The listing builds one solid part. Answer for the finished solid, in the listing's coordinates (mm). A direction names the side the tool comes from. Coordinates: 2 decimals unless noted, no trailing zeros. Order: outer loops, then holes, each group sorted by start corner. A loop starts at its lowest first (then second) coordinate and runs counter-clockwise, first axis right, second up.
```python
from build123d import *

# Parameters (mm, degrees)
F0_W     = 351.6883096945
F0_H     = 200
F1_DEPTH = 25
F2_T     = -2.5
F4_DEPTH = 25


with BuildPart() as f1:
    # F0 (on Front) → F1 (new body)
    with BuildSketch(Plane.XZ):
        with Locations((-175.8441548473, 100)):
            Rectangle(F0_W, F0_H)
    extrude(amount=F1_DEPTH)

    # F2
    f2_openings = [f1.faces().sort_by_distance(p)[0] for p in [
        (-175.844155, -25, 100),
    ]]
    offset(amount=F2_T, openings=f2_openings)

    # F3 (on face) → F4 (join)
    with BuildSketch(Plane.XZ.offset(2.5)):
        Polygon((-291.9401824474, 119.7359256967), (-280.8749377728, 126.1244476883), (-291.9401824474, 132.5129696799), align=None)
        Polygon((-269.8096930981, 106.9588817135), (-269.8096930981, 119.7359256967), (-280.8749377728, 126.1244476883), (-291.9401824474, 119.7359256967), (-291.9401824474, 106.9588817135), (-280.8749377728, 100.570359722), align=None)
        Polygon((-269.8096930981, 119.7359256967), (-269.8096930981, 132.5129696799), (-280.8749377728, 126.1244476883), align=None)
        Polygon((-269.8096930981, 94.1818377304), (-269.8096930981, 106.9588817135), (-280.8749377728, 100.570359722), align=None)
        Polygon((-291.9401824474, 94.1818377304), (-280.8749377728, 100.570359722), (-291.9401824474, 106.9588817135), align=None)
        Polygon((-291.9401824474, 106.9588817135), (-291.9401824474, 119.7359256967), (-303.0054271221, 113.3474037051), align=None)
        Polygon((-258.7444484234, 113.3474037051), (-269.8096930981, 119.7359256967), (-269.8096930981, 106.9588817135), align=None)
    extrude(amount=F4_DEPTH)


solid = f1.part
```
1) Each of these flat-tipped pins is pushed along its axis until it touches: P1, Ø3, axis at x = -172, z = 166, coming from the -Y side; P2, Ø3, axis at x = -240, y = -8, coming from the -Z side. Where does it stop, or does it pass through?
2) A cutting plane is placed at B-B, the plane z = 183. Write down the section's boundary in (x, y), plus the area to 3 significant figures.
3) The mould has two halves that part along Z. Classify faces 3 (the flat face through (-178, -12, 200)), 4 (the flat face through (-291.94, -15, 126)), 5 (the flat face through (-178, 0, 101)): released by +Z, released by -Z, zero draft, split by the parting line, or undercut.
4) A cutting plane is placed at C-C, the plane x = -46. Write down the section's boundary in (y, z), plus the area to 4 significant figures.
5) For faces 1 (the flat face through (-351.688, -12, 99)), 2 (the flat face through (-275.42, -14.82, 97.42)), determine the directions among +Z, -Z, +X, -X, +Y, -Y from which every point of the face is accessible in a straight line to the end or side of a thin tool.
6) Straight lines are drawn through the part: probe 1 along X at (y, z) = (-24.75, 120.5); probe 2 along Z at (x, y) = (-326, -4); probe 3 along X at (y, z) = (-4, 87). For each, find the intervals that lie inside material, in ascending order.
7) A cutting plane is placed at A-A, the plane y = -12.75. Write down the section's boundary in (x, z).
Working result:
1. P1: stops at y = -2.5
1. P2: stops at z = 0
2. outline: (-351.69, -25) - (-349.19, -25) - (-349.19, -2.5) - (-2.5, -2.5) - (-2.5, -25) - (0, -25) - (0, 0) - (-351.69, 0) - close
2. area: 992 mm2
3. face 3: released by +Z
3. face 4: undercut
3. face 5: zero draft
4. outline: (-25, 0) - (0, 0) - (0, 200) - (-25, 200) - (-25, 197.5) - (-2.5, 197.5) - (-2.5, 2.5) - (-25, 2.5) - close
4. area: 612.5 mm2
5. face 1: +Z, -Z, -X, +Y, -Y
5. face 2: -Y
6. probe 1: x = -351.69 to -349.19, -291.94 to -269.81, -2.5 to 0
6. probe 2: z = 0 to 2.5, 197.5 to 200
6. probe 3: x = -351.69 to -349.19, -2.5 to 0
7. outline: (-351.69, 0) - (0, 0) - (0, 200) - (-351.69, 200) - close; (-303.01, 113.35) - (-291.94, 106.96) - (-291.94, 94.18) - (-280.87, 100.57) - (-269.81, 94.18) - (-269.81, 106.96) - (-258.74, 113.35) - (-269.81, 119.74) - (-269.81, 132.51) - (-280.87, 126.12) - (-291.94, 132.51) - (-291.94, 119.74) - close; hole (-349.19, 2.5) - (-2.5, 2.5) - (-2.5, 197.5) - (-349.19, 197.5) - close
